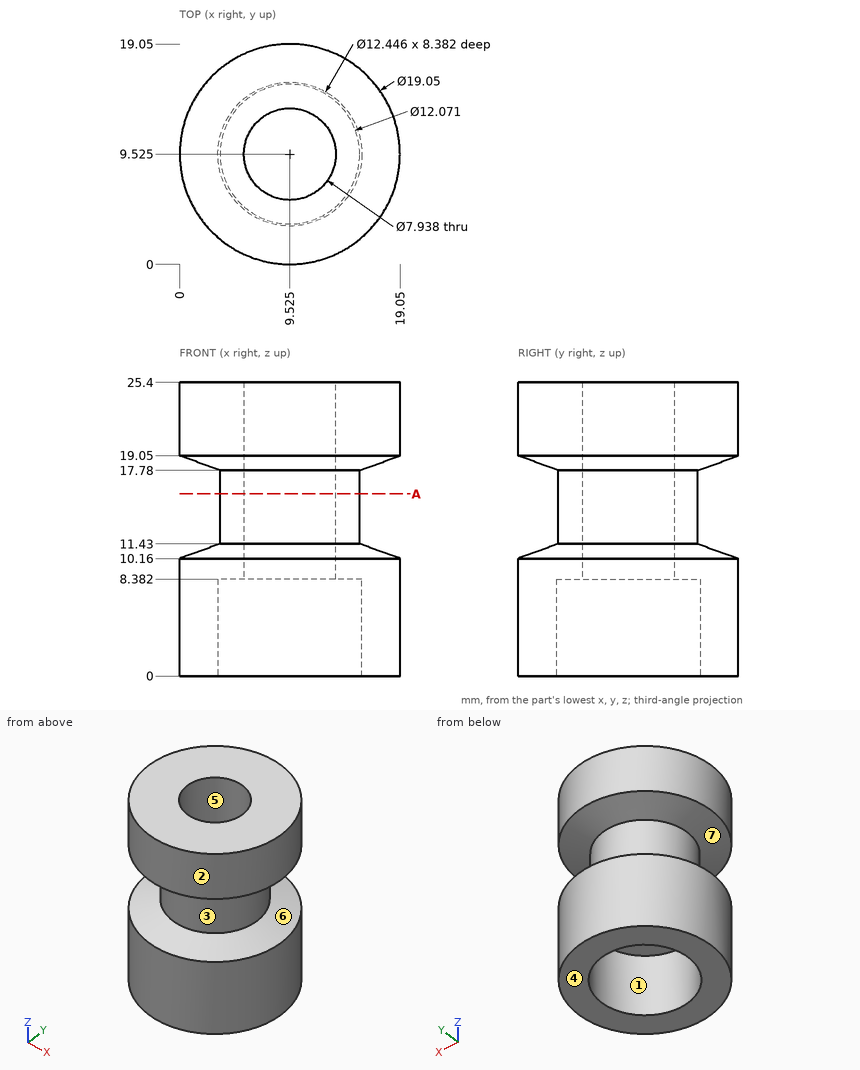
Drawing for the job (mm, zero at the part's lowest x, y, z). A direction names the side the tool comes from. Coordinates: 2 decimals unless noted, no trailing zeros. Order: outer loops, then holes, each group sorted by start corner. A loop starts at its lowest first (then second) coordinate and runs counter-clockwise, first axis right, second up. Notation, with made-up numbers: (-18, -17.75) -> (25, -17.75) arc R6 cw to (25, -8.75) -> close; hole circle Ø1 at (46.25, 15). An arc over 180 degrees is marked (long way). One line per item, written item: value.
(1) Drop flat-ended pins along their axis: pin 1 Ø10 at (x, y) = (9.525, 9.525) entering from -Z; pin 2 Ø3 at (y, z) = (11.5, 19.5) entering from -X; pin 3 Ø3 at (x, z) = (15, 15.5) entering from +Y. Give the stop position or say it passes through.
Checked values:
pin 1: z = 8.38
pin 2: x = 0.01
pin 3: y = 14.07
(2) Mould opens along Z. For the marked faces 4, 5, 6 and 7 say: pulls with the +Z half, pulls with the -Z half, needs draft (parallel to the pull), parting line crosses it, or undercut.
Checked values:
face 4: pulls with the -Z half
face 5: needs draft
face 6: undercut
face 7: undercut
(3) Probe line 1 (Z direction, x = 13.5, y = 8.25); line 2 (Y direction, x = 9.75, z = 22); line 3 (Z direction, x = 12, y = 3.5) (1 decimal). List the from-to ranges inside material, lowest first. Write a range as [from, to].
Checked values:
line 1: [8.38, 25.4]
line 2: [0, 5.56], [13.49, 19.05]
line 3: [0, 11.3], [18, 25.4]
(4) Tool access for the marked faces 1, 2 and 3: list every direction of +Z, -Z, +X, -X, +Y, -Y with a clear straight run to the whole face (end or side of a thin tool).
Checked values:
face 1: -Z
face 2: +Z, -Z
face 3: none
(5) Slice it at A-A, the plane z = 15.75. List the corners of the cut face in (x, y) (1 decimal).
Checked values:
outline: circle Ø12.1 at (9.5, 9.5); hole circle Ø7.9 at (9.5, 9.5)
